Geometry check sheet. Reference: the model listing, model coordinates, mm. Coordinates: 2 decimals unless noted, no trailing zeros. Loops run counter-clockwise (first coordinate to the right, second up) from the corner with the lowest first, then second, coordinate; pieces in that order, holes last.
from build123d import *

# Parameters (mm, degrees)
SKETCH1_R               = 3.81
EXTRUDE1_DEPTH          = 3.937
CHAMFER1_SIZE           = 0.254
CUT_EXTRUDE1_DEPTH      = 7.673242765
CUT_EXTRUDE1_DEPTH_BACK = 7.673242765
SKETCH2_R               = 1.27
CUT_EXTRUDE2_DEPTH      = 7.673242765
CUT_EXTRUDE2_DEPTH_BACK = 7.673242765
SKETCH3_R               = 0.635


with BuildPart() as part:
    # Sketch1 → Extrude1 (new, symmetric)
    with BuildSketch(Plane.XY):
        Circle(SKETCH1_R)
    extrude(amount=EXTRUDE1_DEPTH, both=True)

    # Chamfer1
    chamfer1_edges = [part.edges().sort_by_distance(p)[0] for p in [
        (-3.81, 0, -3.937),
        (-3.81, 0, 3.937),
    ]]
    chamfer(chamfer1_edges, length=CHAMFER1_SIZE)

    # Sketch2 → Cut-Extrude1 (cut, two sides: drawn at the far end of the back side and taken through both)
    with BuildSketch(Plane.XY.offset(-CUT_EXTRUDE1_DEPTH_BACK)):
        Circle(SKETCH2_R)
    extrude(amount=CUT_EXTRUDE1_DEPTH + CUT_EXTRUDE1_DEPTH_BACK, mode=Mode.SUBTRACT)

    # Sketch3 → Cut-Extrude2 (cut, two sides: drawn at the far end of the back side and taken through both)
    with BuildSketch(Plane(origin=(0, 0, 0), x_dir=(1, 0, 0), z_dir=(0, 1, 0)).offset(-CUT_EXTRUDE2_DEPTH_BACK)):
        with Locations(Location((0, 0, 0), (0, 0, 270))):
            Circle(SKETCH3_R)
    extrude(amount=CUT_EXTRUDE2_DEPTH + CUT_EXTRUDE2_DEPTH_BACK, mode=Mode.SUBTRACT)


solid = part.part
1) Section check A-A on y = 0. Record the cut outline in (x, z), and give its area (3 significant figures).
Data:
outline: (-3.81, -3.68) - (-3.56, -3.94) - (-1.27, -3.94) - (-1.27, 3.94) - (-3.56, 3.94) - (-3.81, 3.68) - close; (1.27, -3.94) - (3.56, -3.94) - (3.81, -3.68) - (3.81, 3.68) - (3.56, 3.94) - (1.27, 3.94) - close
area: 39.9 mm2
2) Section check B-B on z = 0. Record the cut outline in (x, y) (3 decimals), and give its area (3 significant figures).
Data:
outline: (-0.635, -3.757) - (-0.635, -1.1) arc R1.27 cw to (-0.635, 1.1) - (-0.635, 3.757) arc R3.81 ccw to start; (0.635, -3.757) arc R3.81 ccw to (0.635, 3.757) - (0.635, 1.1) arc R1.27 cw to (0.635, -1.1) - close
area: 34.0 mm2
3) Mould release check, pull along Z, two halves, no side actions. Record for faces 1 (the flat face through (2, 0, -3.937)), 2 (the cylindrical face through (0.028, 2.436, -0.634)), 3 (the cylindrical face through (-0.936, 0.858, -0.055)): +Z half, -Z half, draft (parallel to the pull), parting line (faces both ways), or undercut.
Data:
face 1: -Z half
face 2: undercut
face 3: draft
4) Material ranges on probe 1 along Z at (x, y) = (0, -3.1) (3 decimals); probe 2 along Y at (x, z) = (0, -1.5); probe 3 along Y at (x, z) = (-0.5, 2), recorded low to high.
Data:
probe 1: z = -3.937 to -0.635, 0.635 to 3.937
probe 2: y = -3.81 to -1.27, 1.27 to 3.81
probe 3: y = -3.78 to -1.17, 1.17 to 3.78
5) Depth check by flat-ended pin: pin 1 (3 mm diameter, centred on x = -2.5, z = -0.5, fed in from +Y); pin 2 (2 mm diameter, centred on x = 2.5, z = 0.5, fed in from +Y); pin 3 (1 mm diameter, centred on y = 1.5, z = -3, fed in from +X); pin 4 (1 mm diameter, centred on x = 0, z = 0, fed in from +Y). Enter the tip coordinate at first touch or a pass-through.
Data:
pin 1: stops at y = 3.68
pin 2: stops at y = 3.5
pin 3: stops at x = 3.68
pin 4: passes through
6) Section check D-D on x = -0.5. Count the separate pieces of the cut face and the enclosed holes in it, and give its area (3 significant figures).
Data:
separate pieces: 4
enclosed holes: 0
area: 36.9 mm2
7) Section check C-C on z = -3. Record the cut outline in (x, y).
Data:
outline: circle Ø7.62 at (0, 0); hole circle Ø2.54 at (0, 0)
